The listing builds one solid part. Answer for the finished solid, in the listing's coordinates (mm). Face numbers are marked on the shaded views. A direction names the side the tool comes from. Round coordinates to 2 decimals unless told otherwise and drop trailing zeros. Write each loop counter-clockwise with the first axis right and the second up, starting at its lowest first coordinate (ties: lowest second). Pieces come first, ordered by that corner, then holes.
(1) Each of these flat-tipped pins is pushed along its axis until it touches: pin 1 Ø1.9 at (y, z) = (3, -2.5) entering from -X; pin 2 Ø2 at (y, z) = (1.5, -2) entering from +X; pin 3 Ø1.4 at (y, z) = (3, -6) entering from +X. Where does it stop, or does it pass through?
(2) Find the intervals of material crossed by probe 1 along X at (y, z) = (1.5, -4.4); probe 2 along X at (y, z) = (3.2, -4.4); probe 3 along Z at (x, y) = (28, 2.2), in increasing order.
(3) A cutting plane is placed at A-A, the plane y = 2.85. Give the vertices of the cut face in (x, z), and give its area (3 significant figures).
(4) A cutting plane is placed at C-C, the plane y = 1.3. Give the vertices of the cut face in (x, z).
(5) The mould has two halves that part along X. Classify the marked faces 1, 2 and 3: +X half, -X half, draft (parallel to the pull), parting line (faces both ways), or undercut.
(6) A cutting plane is placed at D-D, the plane z = -7.5. Give the vertices of the cut face in (x, y).
(7) A cutting plane is placed at B-B, the plane z = -4.4. Give the vertices of the cut face in (x, y).
(8) For the marked faces 4 and 5, determine the directions among +Z, -Z, +X, -X, +Y, -Y from which every point of the face is accessible in a straight line to the end or side of a thin tool.
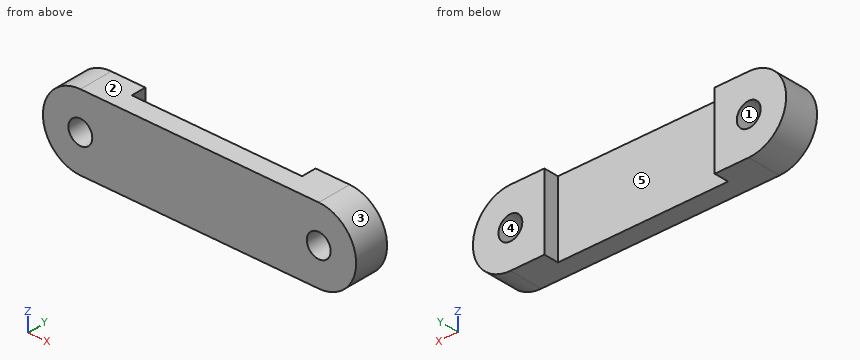
from build123d import *

# Parameters (mm, degrees)
SKETCH1_R           = 1.4
BOSS_EXTRUDE1_DEPTH = 4
SKETCH2_W           = 20
SKETCH2_H           = 8.8
CUT_EXTRUDE1_DEPTH  = 1.75


with BuildPart() as part:
    # Sketch1 → Boss-Extrude1 (new body)
    with BuildSketch(Plane(origin=(0, 0, 0), x_dir=(1, 0, 0), z_dir=(0, 1, 0))):
        with BuildLine():
            Line((0, 0), (28, 0))
            ThreePointArc((28, 0), (32.4, 4.4), (28, 8.8))
            Line((28, 8.8), (0, 8.8))
            ThreePointArc((0, 8.8), (-4.4, 4.4), (0, 0))
        make_face()
        with Locations((0, 4.4)):
            Circle(SKETCH1_R, mode=Mode.SUBTRACT)
        with Locations((28, 4.4)):
            Circle(SKETCH1_R, mode=Mode.SUBTRACT)
    extrude(amount=BOSS_EXTRUDE1_DEPTH)

    # Sketch2 → Cut-Extrude1 (cut)
    with BuildSketch(Plane(origin=(0, 4, 0), x_dir=(1, 0, 0), z_dir=(0, 1, 0))):
        with Locations((14, 4.4)):
            Rectangle(SKETCH2_W, SKETCH2_H)
    extrude(amount=-CUT_EXTRUDE1_DEPTH, mode=Mode.SUBTRACT)


solid = part.part
Solutions:
1. pin 1: stops at x = -4.3
1. pin 2: stops at x = 32.17
1. pin 3: stops at x = 32.31
2. probe 1: x = -4.4 to -1.4, 1.4 to 26.6, 29.4 to 32.4
2. probe 2: x = -4.4 to -1.4, 1.4 to 4, 24 to 26.6, 29.4 to 32.4
2. probe 3: z = -8.8 to -5.8, -3 to 0
3. outline: (0, -8.8) - (4, -8.8) - (4, 0) - (0, 0) arc R4.4 ccw to start; (24, -8.8) - (28, -8.8) arc R4.4 ccw to (28, 0) - (24, 0) - close; hole circle Ø2.8 at (0, -4.4); hole circle Ø2.8 at (28, -4.4)
3. area: 119 mm2
4. outline: (0, -8.8) - (28, -8.8) arc R4.4 ccw to (28, 0) - (0, 0) arc R4.4 ccw to start; hole circle Ø2.8 at (0, -4.4); hole circle Ø2.8 at (28, -4.4)
5. face 1: undercut
5. face 2: draft
5. face 3: +X half
6. outline: (-3.12, 0) - (31.12, 0) - (31.12, 4) - (24, 4) - (24, 2.25) - (4, 2.25) - (4, 4) - (-3.12, 4) - close
7. outline: (-4.4, 0) - (-1.4, 0) - (-1.4, 4) - (-4.4, 4) - close; (1.4, 0) - (26.6, 0) - (26.6, 4) - (24, 4) - (24, 2.25) - (4, 2.25) - (4, 4) - (1.4, 4) - close; (29.4, 0) - (32.4, 0) - (32.4, 4) - (29.4, 4) - close
8. face 4: +Y, -Y
8. face 5: +Z, -Z, +Y
